The model under review builds one solid part; all positions refer to its coordinate system, in mm. A direction names the side the tool comes from. Coordinates: 2 decimals unless noted, no trailing zeros. Order: outer loops, then holes, each group sorted by start corner. A loop starts at its lowest first (then second) coordinate and runs counter-clockwise, first axis right, second up. Notation, with made-up numbers: (-3.5, 1.5) -> (44.5, 1.5) arc R13 ccw to (44.5, 7.5) -> close; hole circle Ø5 at (-20.75, 8.5). An arc over 180 degrees is marked (long way). Use one line per item in the form item = value. Start each with the question number.
(1) Take a section at A-A (z = 12.5). State the section outline as (x, y) points, then the cut area to 3 significant figures.
(2) Mouldability with a two-part tool opening along X and no side actions: class faces 4 (the flat face through (-4, -13.976, 12)), 5 (the cylindrical face through (16.592, -0.411, 20.822)), 6 (the cylindrical face through (-27.329, -1.022, 14.86)), 7 (the cylindrical face through (-3.345, 5.925, 2.465)) as +X half, -X half, draft (parallel to the pull), parting line (faces both ways), or undercut.
(3) Wall thickness on line 1 along X through (y, z) = (-12.45, 12.5); line 2 along X through (y, z) = (-7, 12.5); line 3 along Z through (x, y) = (10.5, 1): over which ranges is each line inside the solid? List them lowest first.
(4) Take a section at D-D (y = -8). State the section outline as (x, z) points, then the cut area to 3 significant figures.
(5) Take a section at B-B (z = 19.75). State the section outline as (x, y) points, then the cut area to 3 significant figures.
(6) Take a section at C-C (x = -4). State the section outline as (y, z) points.
(7) Insertion check: pin 1 Ø10.5 at (x, z) = (16.84, 12.5) entering from -Y; pin 2 Ø4.5 at (x, z) = (16.84, 12.5) entering from -Y; pin 3 Ø4 at (x, y) = (-15, 18) entering from +Z; pin 4 Ø5.5 at (y, z) = (10, 1.5) entering from +X. Each pin has a flat end and moves straight along its axis. Give the tip position at first contact, or say it passes through.
(8) For faces 1 (the flat face through (-5.399, 11, 2)), 2 (the cylindrical face through (-27.656, -6.029, 12.302)), 3 (the cylindrical face through (16.592, -0.411, 6.597)), list the 3-axis set-ups (+Z, -Z, +X, -X, +Y, -Y) from which the entire face can be reached by the end or side of a thin tool; tool diameter is ignored.
```python
from build123d import *

# Parameters (mm, degrees)
EXTRUDE_1_DEPTH     = 25
EXTRUDE_2_DEPTH     = 5
CUT_EXTRUDE_2_DEPTH = 20
FILLET_3_R          = 3.4
FILLET_4_R          = 3.4
SKETCH_5_R          = 2.6
CUT_EXTRUDE_3_DEPTH = 20
SKETCH_7_R          = 4.5
CUT_EXTRUDE_5_DEPTH = 9.98


with BuildPart() as part:
    # Sketch 1 → Extrude 1 (new body)
    with BuildSketch(Plane.XY):
        with BuildLine():
            Line((-24.33363023, 3.038194444), (-28.298611111, 3.038194444))
            Line((-28.298611111, 3.038194444), (-28.298611111, -13.975694444))
            Line((-28.298611111, -13.975694444), (21.701388889, -13.975694444))
            Line((21.701388889, -13.975694444), (21.701388889, 3.038194444))
            Line((21.701388889, 3.038194444), (17.736408008, 3.038194444))
            ThreePointArc((17.736408008, 3.038194444), (-3.298611111, -11.475694444), (-24.33363023, 3.038194444))
        make_face()
    extrude(amount=EXTRUDE_1_DEPTH)

    # Sketch 1_5 → Extrude 2 (add)
    with BuildSketch(Plane.XY):
        with BuildLine():
            Line((17.736408008, 3.038194444), (-24.33363023, 3.038194444))
            ThreePointArc((-24.33363023, 3.038194444), (-3.298611111, -11.475694444), (17.736408008, 3.038194444))
        make_face()
        with BuildLine():
            ThreePointArc((-13.298611111, 21.024305556), (-3.298611111, 25.166441179), (6.701388889, 21.024305556))
            Line((6.701388889, 21.024305556), (21.701388889, 3.038194444))
            Line((21.701388889, 3.038194444), (-28.298611111, 3.038194444))
            Line((-28.298611111, 3.038194444), (-13.298611111, 21.024305556))
        make_face()
        with BuildLine():
            ThreePointArc((-5.398611111, 8.024305556), (-3.298611111, 5.924305556), (-1.198611111, 8.024305556))
            Line((-1.198611111, 8.024305556), (-1.198611111, 14.024305556))
            ThreePointArc((-1.198611111, 14.024305556), (-3.298611111, 16.124305556), (-5.398611111, 14.024305556))
            Line((-5.398611111, 14.024305556), (-5.398611111, 8.024305556))
        make_face(mode=Mode.SUBTRACT)
    extrude(amount=EXTRUDE_2_DEPTH)

    # Sketch 3 → Cut-Extrude 2 (cut)
    with BuildSketch(Plane.XY.offset(25)):
        with BuildLine():
            Line((-28.298611111, 3.038194444), (-28.298611111, 0))
            Line((-28.298611111, 0), (-22.912756186, 0))
            ThreePointArc((-22.912756186, 0), (-23.679884226, 1.492584503), (-24.33363023, 3.038194444))
            Line((-24.33363023, 3.038194444), (-28.298611111, 3.038194444))
        make_face()
        with BuildLine():
            ThreePointArc((17.736408008, 3.038194444), (17.082662004, 1.492584503), (16.315533964, 0))
            Line((16.315533964, 0), (21.701388889, 0))
            Line((21.701388889, 0), (21.701388889, 3.038194444))
            Line((21.701388889, 3.038194444), (17.736408008, 3.038194444))
        make_face()
    extrude(amount=-CUT_EXTRUDE_2_DEPTH, mode=Mode.SUBTRACT)

    # Fillet 3
    fillet_3_edges = [part.edges().sort_by_distance(p)[0] for p in [
        (-28.298611111, 0, 15),
        (-22.912756186, 0, 15),
    ]]
    fillet(fillet_3_edges, radius=FILLET_3_R)

    # Fillet 4
    fillet_4_edges = [part.edges().sort_by_distance(p)[0] for p in [
        (16.315533964, 0, 15),
        (21.701388889, 0, 15),
    ]]
    fillet(fillet_4_edges, radius=FILLET_4_R)

    # Sketch 5 → Cut-Extrude 3 (cut)
    with BuildSketch(Plane(origin=(0, -13.975694444, 0), x_dir=(-1, 0, 0), z_dir=(0, -1, 0))):
        with Locations((23.159932347, -12.5)):
            Circle(SKETCH_5_R)
        with Locations((-16.840067653, -12.5)):
            Circle(SKETCH_5_R)
    extrude(amount=-CUT_EXTRUDE_3_DEPTH, mode=Mode.SUBTRACT)

    # Sketch 7 → Cut-Extrude 5 (cut)
    with BuildSketch(Plane(origin=(0, 0, 0), x_dir=(1, 0, 0), z_dir=(0, 1, 0))):
        with Locations((-23.159932347, -12.5)):
            Circle(SKETCH_7_R)
        with Locations((16.840067653, -12.5)):
            Circle(SKETCH_7_R)
    extrude(amount=-CUT_EXTRUDE_5_DEPTH, mode=Mode.SUBTRACT)


solid = part.part
```
Findings:
q1.outline = (-28.3, -13.98) -> (-25.76, -13.98) -> (-25.76, -9.98) -> (-27.66, -9.98) -> (-27.66, -1.42) arc R3.4 ccw to (-28.3, -3.4) -> close; (-20.56, -13.98) -> (14.24, -13.98) -> (14.24, -9.98) -> (12.34, -9.98) -> (12.34, -5.15) arc R22.5 cw to (-18.66, -5.42) -> (-18.66, -9.98) -> (-20.56, -9.98) -> close; (19.44, -13.98) -> (21.7, -13.98) -> (21.7, -3.4) arc R3.4 ccw to (21.34, -1.87) -> (21.34, -9.98) -> (19.44, -9.98) -> close
q1.area = 180 mm²
q2.face_4 = draft
q2.face_5 = undercut
q2.face_6 = -X half
q2.face_7 = undercut
q3.line_1 = -28.3 to -25.76, -20.56 to 14.24, 19.44 to 21.7
q3.line_2 = -28.3 to -27.66, -18.66 to -16.77, 10.17 to 12.34, 21.34 to 21.7
q3.line_3 = 0 to 5
q4.outline = (-28.3, 0) -> (21.7, 0) -> (21.7, 25) -> (8.71, 25) -> (8.71, 5) -> (-15.31, 5) -> (-15.31, 25) -> (-28.3, 25) -> close; hole circle Ø9 at (-23.16, 12.5); hole circle Ø9 at (16.84, 12.5)
q4.area = 642 mm²
q5.outline = (-28.3, -13.98) -> (21.7, -13.98) -> (21.7, -3.4) arc R3.4 ccw to (18.3, 0) -> (18.21, 0) arc R3.4 ccw to (15.39, -1.51) arc R22.5 cw to (-21.99, -1.51) arc R3.4 ccw to (-24.81, 0) -> (-24.9, 0) arc R3.4 ccw to (-28.3, -3.4) -> close
q5.area = 373 mm²
q6.outline = (-13.98, 0) -> (6.04, 0) -> (6.04, 5) -> (-11.46, 5) -> (-11.46, 25) -> (-13.98, 25) -> close; (16, 0) -> (25.15, 0) -> (25.15, 5) -> (16, 5) -> close
q7.pin_1 = -13.98
q7.pin_2 = through
q7.pin_3 = 5
q7.pin_4 = 18.19
q8.face_1 = +Z, -Z
q8.face_2 = +Y
q8.face_3 = +Z, +Y
